For this review, take the finished solid that the model builds, in its own axes (mm). A direction names the side the tool comes from. Coordinates: 2 decimals unless noted, no trailing zeros. Loops run counter-clockwise (first coordinate to the right, second up) from the corner with the lowest first, then second, coordinate; pieces in that order, holes last. Notation, with made-up numbers: (80.25, 52.25) - (112.25, 52.25) arc R20 cw to (112.25, 79.25) - close; hole circle Ø6 at (-27.5, 20). An arc over 180 degrees is marked (long way). Answer as a JSON object with one key per item and string values. Group by question number.
Item 1: We need section A-A (y = 0). Give the boundary of the cut face in (x, z).
Item 2: We need section C-C (z = 23). Give the boundary of the cut face in (x, y).
Item 3: Tool access review of faces 1 (the flat face through (4, 0, 28)), 2 (the flat face through (0, 4, 28)), 3 (the flat face through (2.5, 8, 11)), 4 (the flat face through (-4, 0, 28)): name each direction out of +Z, -Z, +X, -X, +Y, -Y from which nothing blocks a thin tool from reaching the whole face with its end or side.
Item 4: We need section D-D (x = 1.5). Give the boundary of the cut face in (y, z), then the cut area to 3 significant figures.
Item 5: We need section B-B (x = 0). Give the boundary of the cut face in (y, z), then the cut area to 3 significant figures.
Item 6: To check wall thickness, follow line 1 (Z direction, x = 3.75, y = -5); line 2 (X direction, y = -3.5, z = 34). State the ranges of each line that lie inside material, in increasing order.
Item 7: Clearance check with flat-ended pins moving along their axes: pin 1 (10 mm diameter, centred on y = 7.5, z = 22, fed in from -X); pin 2 (0.8 mm diameter, centred on y = 9, z = 9, fed in from -X); pin 3 (3 mm diameter, centred on x = 0, y = 9, fed in from +Z); pin 4 (8 mm diameter, centred on x = 2, z = 15, fed in from -Y). State where each tip first meets the part, or that it passes through.
from build123d import *

# Parameters (mm, degrees)
SKETCH1_R           = 7.45
BOSS_EXTRUDE1_DEPTH = 21
BOSS_EXTRUDE4_START = -7
SKETCH4_W           = 5
SKETCH4_H           = 9.734089582
BOSS_EXTRUDE4_DEPTH = 8
SKETCH5_W           = 8
SKETCH5_H           = 8
BOSS_EXTRUDE5_DEPTH = 15


with BuildPart() as part:
    # Sketch1 → Boss-Extrude1 (new body)
    with BuildSketch(Plane.XY):
        with Locations(Location((0, 0, 0), (0, 0, 180))):
            Circle(SKETCH1_R)
    extrude(amount=BOSS_EXTRUDE1_DEPTH)

    # Sketch4 → Boss-Extrude4 (add)
    with BuildSketch(Plane(origin=(0, 0, 0), x_dir=(-1, 0, 0), z_dir=(0, 0, -1)).offset(BOSS_EXTRUDE4_START)):
        with Locations((0, 4.867044791)):
            Rectangle(SKETCH4_W, SKETCH4_H)
    extrude(amount=-BOSS_EXTRUDE4_DEPTH)

    # Sketch5 → Boss-Extrude5 (add)
    with BuildSketch(Plane.XY.offset(21)):
        Rectangle(SKETCH5_W, SKETCH5_H)
    extrude(amount=BOSS_EXTRUDE5_DEPTH)


solid = part.part
Check sheet entries:
{
 "1": {"outline": "(-7.45, 0) - (7.45, 0) - (7.45, 21) - (4, 21) - (4, 36) - (-4, 36) - (-4, 21) - (-7.45, 21) - close"},
 "2": {"outline": "(-4, -4) - (4, -4) - (4, 4) - (-4, 4) - close"},
 "3": {"face 1": "+Z, +X, +Y, -Y", "face 2": "+Z, +X, -X, +Y", "face 3": "+Z, -Z, +X, +Y", "face 4": "+Z, -X, +Y, -Y"},
 "4": {"outline": "(-7.3, 0) - (7.3, 0) - (7.3, 7) - (9.73, 7) - (9.73, 15) - (7.3, 15) - (7.3, 21) - (4, 21) - (4, 36) - (-4, 36) - (-4, 21) - (-7.3, 21) - close", "area": "446 mm2"},
 "5": {"outline": "(-7.45, 0) - (7.45, 0) - (7.45, 7) - (9.73, 7) - (9.73, 15) - (7.45, 15) - (7.45, 21) - (4, 21) - (4, 36) - (-4, 36) - (-4, 21) - (-7.45, 21) - close", "area": "451 mm2"},
 "6": {"line 1": "z = 0 to 21", "line 2": "x = -4 to 4"},
 "7": {"pin 1": "stops at x = -6.98", "pin 2": "stops at x = -2.5", "pin 3": "stops at z = 15", "pin 4": "stops at y = -7.45"}
}
